CAD build for the part. Positions are in the model's coordinates, mm. Face numbers are marked on the shaded views. A direction names the side the tool comes from. Give positions to 0.01 mm unless a question says otherwise; leave off trailing zeros. Write each loop counter-clockwise with the first axis right and the second up, starting at its lowest first coordinate (ties: lowest second). Pieces come first, ordered by that corner, then holes. Notation, with made-up numbers: M 86,-12 L 131,-12 A29 ccw 131,23 Z; hole C 16.5,82.5 d7. An arc over 180 degrees is marked long. One line per question, with ' | ' between items. Start each with the question number.
1. Cut at B-B, the plane z = 0. Write the cut outline in (x, y).
2. Cut at D-D, the plane x = 1.75. Write the cut outline in (y, z), then the cut area to 3 significant figures.
3. Cut at C-C, the plane x = 0. Write the cut outline in (y, z).
4. Wall check: L1, parallel to X at y = 4.25, z = 0; L2, parallel to Z at x = -1.25, y = 8.5; L3, parallel to Z at x = -0.75, y = 10.5. Give the ranges that are in metal, low to high.
5. Flat gauge pins, fed straight in: pin 1 (2 mm diameter, centred on x = -2, z = 0, fed in from +Y); pin 2 (3 mm diameter, centred on x = 0.5, z = -1.5, fed in from +Y); pin 3 (1.5 mm diameter, centred on x = 2, y = 11, fed in from -Z). Where does each tip first touch, or does it go through?
6. Which spindle directions (+Z, -Z, +X, -X, +Y, -Y) get a long thin tool onto all of the face, cutting with end or side? Do the marked faces 1 and 2. Say none if no direction does.
7. Cut at A-A, the plane y = 7.5. Write the cut outline in (x, z).
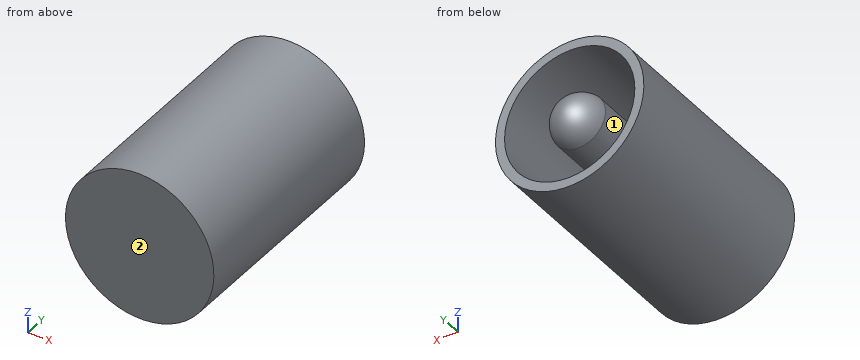
```python
from build123d import *

# Parameters (mm, degrees)
SKETCH1_R           = 4.1671875
BOSS_EXTRUDE1_DEPTH = 12.7
SHELL1_T            = -0.508
SKETCH2_R           = 1.5
BOSS_EXTRUDE2_DEPTH = 11.43
DOME1_FACE_RADIUS   = 1.5
DOME1_HEIGHT        = 1.27


with BuildPart() as part:
    # Sketch1 → Boss-Extrude1 (new body)
    with BuildSketch(Plane(origin=(0, 0, 0), x_dir=(1, 0, 0), z_dir=(0, 1, 0))):
        with Locations(Location((0, 0, 0), (0, 0, 270))):
            Circle(SKETCH1_R)
    extrude(amount=BOSS_EXTRUDE1_DEPTH)

    # Shell1
    shell1_openings = [part.faces().sort_by_distance(p)[0] for p in [
        (0, 12.7, 0),
    ]]
    offset(amount=SHELL1_T, openings=shell1_openings, kind=Kind.INTERSECTION)

    # Sketch2 → Boss-Extrude2 (add)
    with BuildSketch(Plane(origin=(0, 0.508, 0), x_dir=(1, 0, 0), z_dir=(0, 1, 0))):
        with Locations(Location((0, 0, 0), (0, 0, 270))):
            Circle(SKETCH2_R)
    extrude(amount=BOSS_EXTRUDE2_DEPTH)

    # Dome1: a dome of height H over a round flat face of radius A is a cap of a sphere of radius (A * A + H * H) / (2 * H)
    dome1_r = (DOME1_FACE_RADIUS * DOME1_FACE_RADIUS + DOME1_HEIGHT * DOME1_HEIGHT) / (2 * DOME1_HEIGHT)
    dome1_base = Plane((0, 11.938, 0), z_dir=(0, 1, 0))
    with Locations(dome1_base.offset(DOME1_HEIGHT - dome1_r)):
        dome1_ball = Sphere(dome1_r, mode=Mode.PRIVATE)
    add(split(dome1_ball, bisect_by=dome1_base, keep=Keep.TOP, mode=Mode.PRIVATE))


solid = part.part
```
Here are the results:
1) outline: M -4.17,0 L 4.17,0 L 4.17,12.7 L 3.66,12.7 L 3.66,0.51 L 1.5,0.51 L 1.5,11.94 A1.52 ccw -1.5,11.94 L -1.5,0.51 L -3.66,0.51 L -3.66,12.7 L -4.17,12.7 Z
2) outline: M 0,-3.78 L 12.7,-3.78 L 12.7,-3.21 L 0.51,-3.21 L 0.51,3.21 L 12.7,3.21 L 12.7,3.78 L 0,3.78 Z | area: 17.7 mm^2
3) outline: M 0,-4.17 L 12.7,-4.17 L 12.7,-3.66 L 0.51,-3.66 L 0.51,-1.5 L 11.94,-1.5 A1.52 ccw 11.94,1.5 L 0.51,1.5 L 0.51,3.66 L 12.7,3.66 L 12.7,4.17 L 0,4.17 Z
4) L1: -4.17 to -3.66, -1.5 to 1.5, 3.66 to 4.17 | L2: -3.98 to -3.44, -0.83 to 0.83, 3.44 to 3.98 | L3: -4.1 to -3.58, -1.3 to 1.3, 3.58 to 4.1
5) pin 1: y = 12.83 | pin 2: y = 13.21 | pin 3: z = -3.98
6) face 1: +Y | face 2: +Z, -Z, +X, -X, -Y
7) outline: C 0,0 d8.33; C 0,0 d3; hole C 0,0 d7.32
